The model under review builds one solid part; all positions refer to its coordinate system, in mm. A direction names the side the tool comes from. Round coordinates to 2 decimals unless told otherwise and drop trailing zeros. Write each loop counter-clockwise with the first axis right and the second up, starting at its lowest first coordinate (ties: lowest second). Pieces come first, ordered by that corner, then holes. Notation, with made-up numbers: (8.5, -40) -> (26.5, -40) arc R16 ccw to (26.5, -13) -> close; hole circle Ø4 at (-3, 71). An arc over 180 degrees is marked (long way). Answer as a JSON object with one key per item and string values. Group by question number.
1) We need section C-C, the plane x = -23. Write out the cut boundary in (y, z).
2) We need section B-B, the plane z = -42. Write out the cut boundary in (x, y) (3 decimals), then the cut area to 3 significant figures.
3) To check wall thickness, follow probe 1 along Z at (x, y) = (13, -4); probe 2 along X at (y, z) = (-26, -33); probe 3 along X at (y, z) = (-3, -24). State the ranges of each line that lie inside material, in increasing order. Write a range as [from, to].
4) Mouldability with a two-part tool opening along X and no side actions: class faces 1 (the flat face through (-16.998, 12.335, -19.972)), 2 (the cylindrical face through (-10.566, 7.484, -19.972)), 3 (the flat face through (1, -1, -18)) as pulls with the +X half, pulls with the -X half, needs draft (parallel to the pull), parting line crosses it, or undercut.
5) Machinability: for faces 4 (the flat face through (8.617, -23.55, -33.373)), 5 (the cylindrical face through (27.842, -1.212, -28.987)), which of the approach directions +Z, -Z, +X, -X, +Y, -Y give a long, thin tool a straight path to every point of the face, cutting with its end or side? Answer none if there is none.
6) Insertion check: pin 1 Ø5 at (x, y) = (-20, -9.5) entering from -Z; pin 2 Ø1.6 at (x, y) = (7.18, 9.61) entering from +Z; pin 3 Ø4 at (y, z) = (-3, -32.5) entering from -X; pin 4 Ø10 at (x, z) = (-19, -25.5) entering from -Y. Each pin has a flat end and moves straight along its axis. Give the tip position at first contact, or say it passes through.
7) We need section A-A, the plane z = -53. Write out the cut boundary in (x, y).
8) We need section D-D, the plane x = -2. Write out the cut boundary in (y, z).
from build123d import *

# Parameters (mm, degrees)
SKETCH_2_R          = 1
EXTRUDE_1_DEPTH     = 4
SKETCH_5_W          = 42
SKETCH_5_H          = 4
EXTRUDE_2_DEPTH     = 4
EXTRUDE_3_DEPTH     = 42
CUT_EXTRUDE_1_REACH = 94.227
SKETCH_7_R          = 15.5
CUT_EXTRUDE_2_REACH = 94.227
SKETCH_9_R          = 1.5


with BuildPart() as part:
    # 草图2 → 凸台-拉伸1 (new body)
    with BuildSketch(Plane(origin=(0, 0, -18), x_dir=(-1, 0, 0), z_dir=(0, 0, -1))):
        Polygon((-4.251031416, -29.392664593), (29.392664593, -4.251031416), (4.251031416, 29.392664593), (-29.392664593, 4.251031416), align=None)
        with Locations((9.612484574, 7.183323765)):
            Circle(SKETCH_2_R, mode=Mode.SUBTRACT)
        with Locations((-7.183323765, 9.612484574)):
            Circle(SKETCH_2_R, mode=Mode.SUBTRACT)
        with Locations((-9.612484574, -7.183323765)):
            Circle(SKETCH_2_R, mode=Mode.SUBTRACT)
        with Locations((7.183323765, -9.612484574)):
            Circle(SKETCH_2_R, mode=Mode.SUBTRACT)
    extrude(amount=EXTRUDE_1_DEPTH)

    # 草图5 → 凸台-拉伸2 (add)
    with BuildSketch(Plane(origin=(16.821848005, -12.570816589, 0), x_dir=(0.5986103137395574, 0.8010403811822651, 0), z_dir=(0.8010403811822651, -0.5986103137395574, 0))):
        with Locations((0, -20)):
            Rectangle(SKETCH_5_W, SKETCH_5_H)
    extrude(amount=EXTRUDE_2_DEPTH)

    # 草图6 → 凸台-拉伸3 (add)
    with BuildSketch(Plane(origin=(0, 0, -22), x_dir=(-1, 0, 0), z_dir=(0, 0, -1))):
        Polygon((-7.455192941, -31.787105848), (-32.596826118, 1.856590161), (-29.392664593, 4.251031416), (-4.251031416, -29.392664593), align=None)
    extrude(amount=EXTRUDE_3_DEPTH)

    # 草图7 → 切除-拉伸1 (cut, up to next)
    with BuildSketch(Plane(origin=(20.02600953, -14.965257843, 0), x_dir=(-0.5986103137395574, -0.8010403811822653, 0), z_dir=(0.8010403811822653, -0.5986103137395574, 0)), mode=Mode.PRIVATE) as cut_extrude_1_sk1:
        with Locations(Location((0, 43, 0), (0, 0, 180))):
            Circle(SKETCH_7_R)
    cut_extrude_1_tool1 = extrude(cut_extrude_1_sk1.sketch, amount=-CUT_EXTRUDE_1_REACH, mode=Mode.PRIVATE) & part.part
    add(cut_extrude_1_tool1.solids().sort_by_distance((20.02601, -14.965258, -43))[0], mode=Mode.SUBTRACT)

    # 草图9 → 切除-拉伸2 (cut, up to next)
    with BuildSketch(Plane(origin=(20.02600953, -14.965257843, 0), x_dir=(-0.5986103137395573, -0.8010403811822652, 0), z_dir=(0.8010403811822653, -0.5986103137395574, 0)), mode=Mode.PRIVATE) as cut_extrude_2_sk1:
        with Locations(Location((-15.5, 58.5, 0), (0, 0, 180))):
            Circle(SKETCH_9_R)
    cut_extrude_2_tool1 = extrude(cut_extrude_2_sk1.sketch, amount=-CUT_EXTRUDE_2_REACH, mode=Mode.PRIVATE) & part.part
    # 草图9 → 切除-拉伸2 (cut, up to next)
    with BuildSketch(Plane(origin=(20.02600953, -14.965257843, 0), x_dir=(-0.5986103137395573, -0.8010403811822652, 0), z_dir=(0.8010403811822653, -0.5986103137395574, 0)), mode=Mode.PRIVATE) as cut_extrude_2_sk2:
        with Locations((-15.5, 27.5)):
            Circle(SKETCH_9_R)
    cut_extrude_2_tool2 = extrude(cut_extrude_2_sk2.sketch, amount=-CUT_EXTRUDE_2_REACH, mode=Mode.PRIVATE) & part.part
    # 草图9 → 切除-拉伸2 (cut, up to next)
    with BuildSketch(Plane(origin=(20.02600953, -14.965257843, 0), x_dir=(-0.5986103137395573, -0.8010403811822652, 0), z_dir=(0.8010403811822653, -0.5986103137395574, 0)), mode=Mode.PRIVATE) as cut_extrude_2_sk3:
        with Locations((15.5, 58.5)):
            Circle(SKETCH_9_R)
    cut_extrude_2_tool3 = extrude(cut_extrude_2_sk3.sketch, amount=-CUT_EXTRUDE_2_REACH, mode=Mode.PRIVATE) & part.part
    # 草图9 → 切除-拉伸2 (cut, up to next)
    with BuildSketch(Plane(origin=(20.02600953, -14.965257843, 0), x_dir=(-0.5986103137395573, -0.8010403811822652, 0), z_dir=(0.8010403811822653, -0.5986103137395574, 0)), mode=Mode.PRIVATE) as cut_extrude_2_sk4:
        with Locations(Location((15.5, 27.5, 0), (0, 0, 180))):
            Circle(SKETCH_9_R)
    cut_extrude_2_tool4 = extrude(cut_extrude_2_sk4.sketch, amount=-CUT_EXTRUDE_2_REACH, mode=Mode.PRIVATE) & part.part
    add(cut_extrude_2_tool1.solids().sort_by_distance((29.304469, -2.549132, -58.5))[0], mode=Mode.SUBTRACT)
    add(cut_extrude_2_tool2.solids().sort_by_distance((29.304469, -2.549132, -27.5))[0], mode=Mode.SUBTRACT)
    add(cut_extrude_2_tool3.solids().sort_by_distance((10.74755, -27.381384, -58.5))[0], mode=Mode.SUBTRACT)
    add(cut_extrude_2_tool4.solids().sort_by_distance((10.74755, -27.381384, -27.5))[0], mode=Mode.SUBTRACT)


solid = part.part
Here are the results:
{
 "1": {"outline": "(-9.03, -22) -> (4.3, -22) -> (4.3, -18) -> (-9.03, -18) -> close"},
 "2": {"outline": "(4.251, -29.393) -> (7.455, -31.787) -> (10.767, -27.356) -> (7.563, -24.961) -> close; (26.081, -0.181) -> (29.285, -2.575) -> (32.597, 1.857) -> (29.393, 4.251) -> close", "area": "44.3 mm^2"},
 "3": {"probe 1": "z = [-22, -18]", "probe 2": "x = [6.79, 11.78]", "probe 3": "x = [23.97, 28.97]"},
 "4": {"face 1": "pulls with the -X half", "face 2": "undercut", "face 3": "needs draft"},
 "5": {"face 4": "-Z, -X, +Y", "face 5": "none"},
 "6": {"pin 1": "stops at z = -22", "pin 2": "passes through", "pin 3": "stops at x = 22.84", "pin 4": "stops at y = -14.69"},
 "7": {"outline": "(4.25, -29.39) -> (7.46, -31.79) -> (12.94, -24.45) -> (9.73, -22.06) -> close; (23.91, -3.08) -> (27.12, -5.48) -> (32.6, 1.86) -> (29.39, 4.25) -> close"},
 "8": {"outline": "(-24.72, -22) -> (27.71, -22) -> (27.71, -18) -> (-24.72, -18) -> close"}
}
